Part model, mm, in its own coordinate system. Face numbers are marked on the shaded views. A direction names the side the tool comes from. Give positions to 0.01 mm unless a question says otherwise; leave off trailing zeros. Order: outer loops, then holes, each group sorted by start corner. A loop starts at its lowest first (then second) coordinate and runs counter-clockwise, first axis right, second up. Notation, with made-up numbers: M 67.5,55 L 71.5,55 A12 ccw 71.5,72 Z; hole C 87.25,39.25 d9. An arc over 180 degrees is marked long. Answer as a JSON object with one key per item and string values.
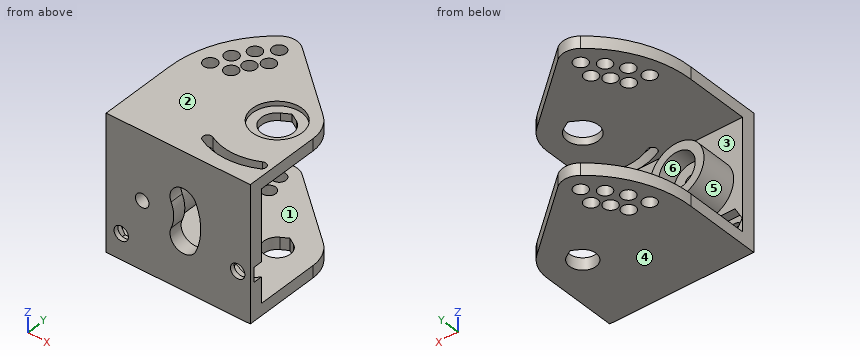
from build123d import *

# Parameters (mm, degrees)
SKETCH1_R           = 6
BOSS_EXTRUDE1_DEPTH = 3
SKETCH1_3_R         = 1.6
BOSS_EXTRUDE5_DEPTH = 1
SKETCH1_6_R         = 6
SKETCH1_6_R_2       = 4.05
BOSS_EXTRUDE6_DEPTH = 11
SKETCH1_7_R         = 4.05
SKETCH1_7_R_2       = 1.5
BOSS_EXTRUDE7_DEPTH = 7
SKETCH2_R           = 1.5
BOSS_EXTRUDE2_DEPTH = 2.666
CUT_EXTRUDE1_DEPTH  = 2.666
CUT_EXTRUDE2_DEPTH  = 2.666
SKETCH3_3_R         = 5.5
CUT_EXTRUDE4_DEPTH  = 1


with BuildPart() as part:
    # Sketch1 → Boss-Extrude1 (new body)
    with BuildSketch(Plane(origin=(0, 0, 0), x_dir=(1, 0, 0), z_dir=(0, 1, 0))):
        Polygon((0, 15), (0, -15), (32, -15), (32, 3.383419246), (29.2, 1.766838493), (26.4, 3.383419246), (26.4, 6.616580754), (29.2, 8.233161507), (32, 6.616580754), (32, 15), align=None)
        with Locations(Location((8, 0, 0), (0, 0, 270))):
            Circle(SKETCH1_R, mode=Mode.SUBTRACT)
        with BuildLine():
            ThreePointArc((19.914696807, 5.2), (21, 0), (19.914696807, -5.2))
            ThreePointArc((19.914696807, -5.2), (15.96515139, -6.749545417), (14.415605973, -2.8))
            ThreePointArc((14.415605973, -2.8), (15, 0), (14.415605973, 2.8))
            ThreePointArc((14.415605973, 2.8), (15.96515139, 6.749545417), (19.914696807, 5.2))
        make_face(mode=Mode.SUBTRACT)
        Polygon((6.566323015, 9.3334), (4.949742261, 6.5334), (1.716580754, 6.5334), (0.1, 9.3334), (1.716580754, 12.1334), (4.949742261, 12.1334), align=None, mode=Mode.SUBTRACT)
    extrude(amount=BOSS_EXTRUDE1_DEPTH)

    # Sketch1<3> → Boss-Extrude5 (add)
    # profile 1 of 2: a face of its own
    with BuildSketch(Plane(origin=(0, 0, 0), x_dir=(1, 0, 0), z_dir=(0, 1, 0))):
        Polygon((29.2, 1.766838493), (32, 3.383419246), (32, 6.616580754), (29.2, 8.233161507), (26.4, 6.616580754), (26.4, 3.383419246), align=None)
        with Locations(Location((29.2, 5, 0), (0, 0, 270))):
            Circle(SKETCH1_3_R, mode=Mode.SUBTRACT)
    # profile 2 of 2: a face of its own
    with BuildSketch(Plane(origin=(0, 0, 0), x_dir=(1, 0, 0), z_dir=(0, 1, 0))):
        Polygon((1.716580754, 6.5334), (4.949742261, 6.5334), (6.566323015, 9.3334), (4.949742261, 12.1334), (1.716580754, 12.1334), (0.1, 9.3334), align=None)
        with Locations(Location((3.333161507, 9.3334, 0), (0, 0, 270))):
            Circle(SKETCH1_3_R, mode=Mode.SUBTRACT)
    extrude(amount=BOSS_EXTRUDE5_DEPTH)

    # Sketch1<6> → Boss-Extrude6 (add)
    with BuildSketch(Plane(origin=(0, 0, 0), x_dir=(1, 0, 0), z_dir=(0, 1, 0))):
        with Locations(Location((8, 0, 0), (0, 0, 270))):
            Circle(SKETCH1_6_R)
        with Locations(Location((8, 0, 0), (0, 0, 270))):
            Circle(SKETCH1_6_R_2, mode=Mode.SUBTRACT)
    extrude(amount=BOSS_EXTRUDE6_DEPTH)

    # Sketch1<7> → Boss-Extrude7 (add)
    with BuildSketch(Plane(origin=(0, 0, 0), x_dir=(1, 0, 0), z_dir=(0, 1, 0))):
        with Locations(Location((8, 0, 0), (0, 0, 270))):
            Circle(SKETCH1_7_R)
        with Locations(Location((8, 0, 0), (0, 0, 270))):
            Circle(SKETCH1_7_R_2, mode=Mode.SUBTRACT)
    extrude(amount=BOSS_EXTRUDE7_DEPTH)

    # Sketch2 → Boss-Extrude2 (add)
    with BuildSketch(Plane.XY.offset(15)):
        with BuildLine():
            ThreePointArc((32, 17), (31.250462296, 20.380946094), (29.142300877, 23.128355545))
            Line((29.142300877, 23.128355545), (14.13095683, 35.724368799))
            ThreePointArc((14.13095683, 35.724368799), (11.613454774, 36.659831241), (9.07176767, 35.792229231))
            ThreePointArc((9.07176767, 35.792229231), (2.386606283, 27.433657654), (0, 17))
            Line((0, 17), (0, 3))
            Line((0, 3), (32, 3))
            Line((32, 3), (32, 17))
        make_face()
        with Locations((4.730842624, 22.357198336)):
            Circle(SKETCH2_R, mode=Mode.SUBTRACT)
        with Locations((6.265744109, 26.24641379)):
            Circle(SKETCH2_R, mode=Mode.SUBTRACT)
        with Locations((8.86645275, 22.972542385)):
            Circle(SKETCH2_R, mode=Mode.SUBTRACT)
        with Locations((10.438918453, 25.988469401)):
            Circle(SKETCH2_R, mode=Mode.SUBTRACT)
        with Locations((8.575717674, 29.731516592)):
            Circle(SKETCH2_R, mode=Mode.SUBTRACT)
        with Locations((12.604068492, 28.611557173)):
            Circle(SKETCH2_R, mode=Mode.SUBTRACT)
        with Locations((11.559806391, 32.660191026)):
            Circle(SKETCH2_R, mode=Mode.SUBTRACT)
    boss_extrude2 = extrude(amount=-BOSS_EXTRUDE2_DEPTH)

    # Mirror1: Boss-Extrude2 across plane
    add(boss_extrude2.mirror(Plane.XY))

    # Sketch3 → Cut-Extrude1 (cut)
    with BuildSketch(Plane.XY.offset(15)):
        with BuildLine():
            Line((22.25, 20.031088913), (24, 21.041451884))
            Line((24, 21.041451884), (25.75, 20.031088913))
            ThreePointArc((25.75, 20.031088913), (24, 13.5), (22.25, 20.031088913))
        make_face()
        with BuildLine():
            ThreePointArc((18.461538462, 6.354557605), (24, 5), (29.538461538, 6.354557605))
            ThreePointArc((29.538461538, 6.354557605), (30.8871202, 5.928975867), (30.461538462, 4.580317206))
            ThreePointArc((30.461538462, 4.580317206), (24, 3), (17.538461538, 4.580317206))
            ThreePointArc((17.538461538, 4.580317206), (17.1128798, 5.928975867), (18.461538462, 6.354557605))
        make_face()
    extrude(amount=-CUT_EXTRUDE1_DEPTH, mode=Mode.SUBTRACT)

    # Sketch4 → Cut-Extrude2 (cut)
    with BuildSketch(Plane.XY.offset(-12.334)):
        with BuildLine():
            Line((22.5275, 19.550444814), (24, 20.400593086))
            Line((24, 20.400593086), (25.4725, 19.550444814))
            ThreePointArc((25.4725, 19.550444814), (24, 14.055), (22.5275, 19.550444814))
        make_face()
    extrude(amount=-CUT_EXTRUDE2_DEPTH, mode=Mode.SUBTRACT)

    # Sketch3<3> → Cut-Extrude4 (cut)
    # profile 1 of 2: a face of its own
    with BuildSketch(Plane.XY.offset(15)):
        with Locations((24, 17)):
            Circle(SKETCH3_3_R)
        with BuildLine():
            Line((22.25, 20.031088913), (24, 21.041451884))
            Line((24, 21.041451884), (25.75, 20.031088913))
            ThreePointArc((25.75, 20.031088913), (24, 13.5), (22.25, 20.031088913))
        make_face(mode=Mode.SUBTRACT)
    # profile 2 of 2: a face of its own
    with BuildSketch(Plane.XY.offset(15)):
        with BuildLine():
            ThreePointArc((17.538461538, 4.580317206), (24, 3), (30.461538462, 4.580317206))
            ThreePointArc((30.461538462, 4.580317206), (30.8871202, 5.928975867), (29.538461538, 6.354557605))
            ThreePointArc((29.538461538, 6.354557605), (24, 5), (18.461538462, 6.354557605))
            ThreePointArc((18.461538462, 6.354557605), (17.1128798, 5.928975867), (17.538461538, 4.580317206))
        make_face()
    extrude(amount=-CUT_EXTRUDE4_DEPTH, mode=Mode.SUBTRACT)


solid = part.part
1. Cut at A-A on x = 18. Give the cut face in (y, z).
Worked answers:
{"outline": "M 0,-15 L 32.48,-15 L 32.48,-12.33 L 3,-12.33 L 3,-6.88 L 0,-6.88 Z; M 0,6.88 L 3,6.88 L 3,12.33 L 4.35,12.33 L 4.35,15 L 0,15 Z; M 6.47,12.33 L 32.48,12.33 L 32.48,15 L 6.47,15 Z"}
2. Cut at C-C on z = 9. Give the cut face in (x, y).
Worked answers:
{"outline": "M 0,0 L 32,0 L 32,3 L 0,3 Z"}
3. Probe line 1 along Z through (x, y) = (23, 7.5); line 2 along Z through (x, y) = (10.5, 10.5); line 3 along Y through (x, z) = (23, -6.5). List the from-to ranges inside material, lowest first.
Worked answers:
{"line 1": "z = -15 to -12.33, 12.33 to 15", "line 2": "z = -15 to -12.33, -5.45 to -3.19, 3.19 to 5.45, 12.33 to 15", "line 3": "y = 0 to 3"}
4. Cut at B-B on x = 23. State how many separate pieces and enclosed holes the cut face has, plus the area to 3 significant figures.
Worked answers:
{"separate pieces": "4", "enclosed holes": "0", "area": "182 mm^2"}
5. Two-plate mould, pull along X, no slides. Class the marked faces 4, 5 and 6: +X half, -X half, draft (parallel to the pull), parting line (faces both ways), or undercut.
Worked answers:
{"face 4": "draft", "face 5": "parting line", "face 6": "undercut"}
6. Which spindle directions (+Z, -Z, +X, -X, +Y, -Y) get a long thin tool onto all of the face, cutting with end or side? Do the marked faces 1, 2 and 3. Say none if no direction does.
Worked answers:
{"face 1": "+X, -X, +Y", "face 2": "+Z, +X, -X, +Y, -Y", "face 3": "+Y"}
7. Pin check, flat tips, straight feed: P1, Ø10, axis at y = 22, z = -11, coming from the +X side; P2, Ø4.5, axis at x = 4, z = -8.5, coming from the +Y side; P3, Ø6.5, axis at x = 7, z = -0.5, coming from the +Y side. Stop position of each tip, or through.
Worked answers:
{"P1": "stops at x = 32", "P2": "stops at y = 3", "P3": "stops at y = 11"}
8. Cut at D-D on x = 30. Give the cut face in (y, z), plus the area to 3 significant figures.
Worked answers:
{"outline": "M 0,-15 L 22.29,-15 L 22.29,-12.33 L 3,-12.33 L 3,-7.77 L 1,-7.77 L 1,-6.39 L 0,-6.39 Z; M 0,-3.61 L 1,-3.61 L 1,-2.23 L 3,-2.23 L 3,12.33 L 4.35,12.33 L 4.35,15 L 0,15 Z; M 6.47,12.33 L 22.29,12.33 L 22.29,15 L 6.47,15 Z", "area": "173 mm^2"}
